Here's how the part is built. I have some questions about the finished solid (model axes, mm). A direction names the side the tool comes from. Round coordinates to 2 decimals unless told otherwise and drop trailing zeros. Order: outer loops, then holes, each group sorted by start corner. A loop starts at its lowest first (then second) coordinate and runs counter-clockwise, first axis right, second up. Notation, with made-up numbers: (50.25, 20.5) -> (90.25, 20.5) arc R34 cw to (90.25, 54.5) -> close; hole circle Ø5 at (65.5, 58.25). An arc over 180 degrees is marked (long way). Answer in a Markdown table with one row per item.
```python
from build123d import *

# Parameters (mm, degrees)
SKETCH1_W            = 203.2
SKETCH1_H            = 101.6
BOSS_EXTRUDE1_DEPTH  = 5.08
SKETCH2_W            = 167.467297736
SKETCH2_H            = 13.584196144
CUT_EXTRUDE4_DEPTH   = 114.705788771
BOSS_EXTRUDE2_DEPTH  = 21.59
FILLET1_R            = 2.54
FILLET2_R            = 2.54
MIRROR3_COPY_1_DEPTH = 21.59
FILLET3_R            = 2.54
SKETCH5_W            = 64.377921573
SKETCH5_H            = 57.58977338
BOSS_EXTRUDE4_DEPTH  = 20.32
SKETCH6_W            = 59.998471125
SKETCH6_H            = 52.334432844
CUT_EXTRUDE5_DEPTH   = 20.32
SKETCH7_W            = 37.334815061
SKETCH7_H            = 5.20069898
CUT_EXTRUDE6_DEPTH   = 124.024580753
SKETCH8_W            = 45.765257173
SKETCH8_H            = 5.912359678
CUT_EXTRUDE7_DEPTH   = 132.792241377
FILLET4_R            = 2.54


with BuildPart() as part:
    # Sketch1 → Boss-Extrude1 (new body)
    with BuildSketch(Plane(origin=(0, 0, 0), x_dir=(1, 0, 0), z_dir=(0, 1, 0))):
        Rectangle(SKETCH1_W, SKETCH1_H)
    extrude(amount=BOSS_EXTRUDE1_DEPTH)

    # Sketch2 → Cut-Extrude4 (cut, through all)
    with BuildSketch(Plane(origin=(0, 5.08, 0), x_dir=(1, 0, 0), z_dir=(0, 1, 0))):
        Polygon((83.693773799, 50.8), (-83.82, 50.8), (-83.82, 50.443396551), (-83.82, 38.767661401), (83.693773799, 38.767661401), (83.693773799, 50.443396551), align=None)
        with BuildLine():
            Line((101.6, 50.8), (83.82, 50.8))
            ThreePointArc((83.82, 50.8), (96.392358569, 45.592358569), (101.6, 33.02))
            Line((101.6, 33.02), (101.6, 50.8))
        make_face()
        with BuildLine():
            Line((101.6, -50.8), (101.6, -33.02))
            ThreePointArc((101.6, -33.02), (96.392358569, -45.592358569), (83.82, -50.8))
            Line((83.82, -50.8), (101.6, -50.8))
        make_face()
        with BuildLine():
            ThreePointArc((-84.074, -50.8), (-96.466753447, -45.666753447), (-101.6, -33.274))
            Line((-101.6, -33.274), (-101.6, -50.8))
            Line((-101.6, -50.8), (-84.074, -50.8))
        make_face()
        with BuildLine():
            ThreePointArc((-101.6, 33.274), (-96.466753447, 45.666753447), (-84.074, 50.8))
            Line((-84.074, 50.8), (-101.6, 50.8))
            Line((-101.6, 50.8), (-101.6, 33.274))
        make_face()
        with Locations((-0.086351132, -44.007901928)):
            Rectangle(SKETCH2_W, SKETCH2_H)
    extrude(amount=-CUT_EXTRUDE4_DEPTH, mode=Mode.SUBTRACT)

    # Sketch4 → Boss-Extrude2 (add)
    with BuildSketch(Plane(origin=(0, 5.08, 0), x_dir=(1, 0, 0), z_dir=(0, 1, 0))):
        Polygon((-83.82, 16.161661401), (-17.736774311, 16.161661401), (-17.736774311, 38.767661401), (-20.145472057, 38.767661401), (-20.145472057, 18.447661401), (-83.82, 18.447661401), align=None)
    boss_extrude2 = extrude(amount=BOSS_EXTRUDE2_DEPTH)

    # Fillet1
    fillet1_edges = [part.edges().sort_by_distance(p)[0] for p in [
        (-17.736774311, 15.875, -16.161661401),
    ]]
    fillet(fillet1_edges, radius=FILLET1_R)

    # Mirror1: Boss-Extrude2 across plane
    add(boss_extrude2.mirror(Plane(origin=(0, 0, 0), x_dir=(0, 0, 1), z_dir=(1, 0, 0))))

    # Fillet2
    fillet2_edges = [part.edges().sort_by_distance(p)[0] for p in [
        (17.736774311, 15.875, -16.161661401),
    ]]
    fillet(fillet2_edges, radius=FILLET2_R)

    # Mirror3: Boss-Extrude2 across plane
    add(boss_extrude2.mirror(Plane.XY))

    # Mirror3 copy 1 sketch → Mirror3 copy 1 (add)
    with BuildSketch(Plane(origin=(0, 5.08, 0), x_dir=(-1, 0, 0), z_dir=(0, 1, 0))):
        Polygon((-83.82, 16.161661401), (-17.736774311, 16.161661401), (-17.736774311, 38.767661401), (-20.145472057, 38.767661401), (-20.145472057, 18.447661401), (-83.82, 18.447661401), align=None)
    extrude(amount=MIRROR3_COPY_1_DEPTH)

    # Fillet3
    fillet3_edges = [part.edges().sort_by_distance(p)[0] for p in [
        (-17.736774311, 15.875, 16.161661401),
        (17.736774311, 15.875, 16.161661401),
    ]]
    fillet(fillet3_edges, radius=FILLET3_R)

    # Sketch5 → Boss-Extrude4 (add)
    with BuildSketch(Plane.XZ):
        with Locations((39.415054025, 0)):
            Rectangle(SKETCH5_W, SKETCH5_H)
    extrude(amount=BOSS_EXTRUDE4_DEPTH)

    # Sketch6 → Cut-Extrude5 (cut)
    with BuildSketch(Plane.XZ.offset(20.32)):
        with Locations((39.634026547, 0)):
            Rectangle(SKETCH6_W, SKETCH6_H)
    extrude(amount=-CUT_EXTRUDE5_DEPTH, mode=Mode.SUBTRACT)

    # Sketch7 → Cut-Extrude6 (cut, through all)
    with BuildSketch(Plane.ZY.offset(-7.226093238)):
        with Locations((0.602174437, -2.60034949)):
            Rectangle(SKETCH7_W, SKETCH7_H)
    extrude(amount=-CUT_EXTRUDE6_DEPTH, mode=Mode.SUBTRACT)

    # Sketch8 → Cut-Extrude7 (cut, through all)
    with BuildSketch(Plane(origin=(0, 0, -28.79488669), x_dir=(-1, 0, 0), z_dir=(0, 0, -1))):
        with Locations((-39.524540286, -2.956179839)):
            Rectangle(SKETCH8_W, SKETCH8_H)
    extrude(amount=-CUT_EXTRUDE7_DEPTH, mode=Mode.SUBTRACT)

    # Fillet4
    fillet4_edges = [part.edges().sort_by_distance(p)[0] for p in [
        (7.226093238, -10.16, 28.79488669),
        (7.226093238, -10.16, -28.79488669),
        (71.604014811, -10.16, -28.79488669),
        (71.604014811, -10.16, 28.79488669),
    ]]
    fillet(fillet4_edges, radius=FILLET4_R)


solid = part.part
```
1. Suppose I cut it at A-A on y = 9. Write out the boundary of the cut face in (x, z), then the cut area to 3 significant figures.
Numbers:
| item | result |
|---|---|
| outline | (-83.82, -18.45) -> (-20.15, -18.45) -> (-20.15, -38.77) -> (-17.74, -38.77) -> (-17.74, -18.7) arc R2.54 ccw to (-20.28, -16.16) -> (-83.82, -16.16) -> close; (-83.82, 16.16) -> (-20.28, 16.16) arc R2.54 ccw to (-17.74, 18.7) -> (-17.74, 38.77) -> (-20.15, 38.77) -> (-20.15, 18.45) -> (-83.82, 18.45) -> close; (17.74, -38.77) -> (20.15, -38.77) -> (20.15, -18.45) -> (83.82, -18.45) -> (83.82, -16.16) -> (20.28, -16.16) arc R2.54 ccw to (17.74, -18.7) -> close; (17.74, 18.7) arc R2.54 ccw to (20.28, 16.16) -> (83.82, 16.16) -> (83.82, 18.45) -> (20.15, 18.45) -> (20.15, 38.77) -> (17.74, 38.77) -> close |
| area | 795 mm2 |
2. Suppose I cut it at D-D on x = -61.5. Write out the boundary of the cut face in (y, z).
Numbers:
| item | result |
|---|---|
| outline | (0, -38.77) -> (5.08, -38.77) -> (5.08, -18.45) -> (26.67, -18.45) -> (26.67, -16.16) -> (5.08, -16.16) -> (5.08, 16.16) -> (26.67, 16.16) -> (26.67, 18.45) -> (5.08, 18.45) -> (5.08, 37.22) -> (0, 37.22) -> close |
3. For faces 1 (the face through (9.635, -13, 0)), 2 (the face through (52, 16, 18.448)), 3 (the face through (20.145, 16, -29)), which set-ups out of +Z, -Z, +X, -X, +Y, -Y let a thin tool reach every point of the face, with its end or its side?
Numbers:
| item | result |
|---|---|
| face 1 | -Y |
| face 2 | +Z, +X, +Y |
| face 3 | -Z, +X, +Y |
4. Suppose I cut it at C-C on y = -16.5. Write out the boundary of the cut face in (x, z), then the cut area to 3 significant figures.
Numbers:
| item | result |
|---|---|
| outline | (7.23, -26.25) arc R2.54 ccw to (9.77, -28.79) -> (69.06, -28.79) arc R2.54 ccw to (71.6, -26.25) -> (71.6, 26.25) arc R2.54 ccw to (69.06, 28.79) -> (9.77, 28.79) arc R2.54 ccw to (7.23, 26.25) -> close; hole (9.63, -26.17) -> (69.63, -26.17) -> (69.63, 26.17) -> (9.63, 26.17) -> close |
| area | 562 mm2 |
5. Please list where these lines run through material, in increasing order: line 1 along X through (y, z) = (12, -23.5); line 2 along Z through (x, y) = (21, -14); line 3 along Z through (x, y) = (74, 16).
Numbers:
| item | result |
|---|---|
| line 1 | x = -20.15 to -17.74, 17.74 to 20.15 |
| line 2 | z = -28.79 to -26.17, 26.17 to 28.79 |
| line 3 | z = -18.45 to -16.16, 16.16 to 18.45 |
6. We'd pull the mould along Z, two halves only. Please class faces 4 (the face through (-52, 16, -16.162)), 5 (the face through (96.253, 2.576, -45.73)), 6 (the face through (37, -20.32, -28)), 7 (the face through (-52, 16, 16.162)): released by +Z, released by -Z, zero draft, split by the parting line, or undercut.
Numbers:
| item | result |
|---|---|
| face 4 | undercut |
| face 5 | released by -Z |
| face 6 | zero draft |
| face 7 | undercut |
7. For pin 1 Ø12 at (y, z) = (-10.5, 14) entering from -X; pin 2 Ø1.5 at (x, z) = (-23.5, 1) entering from +Y; pin 3 Ø4 at (y, z) = (3, -42) entering from +X; pin 4 Ø5 at (y, z) = (-4, -36) entering from +X, each with a flat end and sliding along its axis, tell me the tip position at first contact or that it passes through.
Numbers:
| item | result |
|---|---|
| pin 1 | stops at x = 7.23 |
| pin 2 | stops at y = 5.08 |
| pin 3 | stops at x = 100.17 |
| pin 4 | passes through |
8. Suppose I cut it at B-B on z = 8.5. Write out the boundary of the cut face in (x, y), then the cut area to 3 significant figures.
Numbers:
| item | result |
|---|---|
| outline | (-101.6, 0) -> (101.6, 0) -> (101.6, 5.08) -> (-101.6, 5.08) -> close; (7.23, -20.32) -> (9.63, -20.32) -> (9.63, -5.2) -> (7.23, -5.2) -> close; (69.63, -20.32) -> (71.6, -20.32) -> (71.6, -5.2) -> (69.63, -5.2) -> close |
| area | 1,100 mm2 |
